```python
from build123d import *

# Parameters (mm, degrees)
SKETCH1_W           = 95
SKETCH1_H           = 75
BOSS_EXTRUDE1_DEPTH = 2
SKETCH2_W           = 14
SKETCH2_H           = 4
SKETCH2_W_2         = 13
BOSS_EXTRUDE2_DEPTH = 4
SKETCH3_W           = 12
SKETCH3_H           = 4
SKETCH3_W_2         = 11
BOSS_EXTRUDE3_DEPTH = 250
SKETCH4_W           = 10
SKETCH4_H           = 4
SKETCH4_W_2         = 9
BOSS_EXTRUDE4_DEPTH = 4
SKETCH5_W           = 4
SKETCH5_H           = 15
BOSS_EXTRUDE5_DEPTH = 4
SKETCH6_W           = 20
SKETCH6_H           = 4
BOSS_EXTRUDE6_DEPTH = 4


with BuildPart() as part:
    # Sketch1 → Boss-Extrude1 (new, symmetric)
    with BuildSketch(Plane.XY):
        Rectangle(SKETCH1_W, SKETCH1_H)
    extrude(amount=BOSS_EXTRUDE1_DEPTH, both=True)

    # Sketch2 → Boss-Extrude2 (add)
    with BuildSketch(Plane(origin=(0, 37.5, 0), x_dir=(1, 0, 0), z_dir=(0, 1, 0))):
        with Locations((40.5, 0)):
            Rectangle(SKETCH2_W, SKETCH2_H)
        with Locations((21, 0)):
            Rectangle(SKETCH2_W_2, SKETCH2_H)
        with Locations((-40.5, 0)):
            Rectangle(SKETCH2_W, SKETCH2_H)
        with Locations((-21, 0)):
            Rectangle(SKETCH2_W_2, SKETCH2_H)
    extrude(amount=BOSS_EXTRUDE2_DEPTH)

    # Sketch3 → Boss-Extrude3 (add)
    with BuildSketch(Plane(origin=(0, 41.5, 0), x_dir=(1, 0, 0), z_dir=(0, 1, 0))):
        with Locations((41.5, 0)):
            Rectangle(SKETCH3_W, SKETCH3_H)
        with Locations((22, 0)):
            Rectangle(SKETCH3_W_2, SKETCH3_H)
        with Locations((-22, 0)):
            Rectangle(SKETCH3_W_2, SKETCH3_H)
        with Locations((-41.5, 0)):
            Rectangle(SKETCH3_W, SKETCH3_H)
    extrude(amount=BOSS_EXTRUDE3_DEPTH)

    # Sketch4 → Boss-Extrude4 (add)
    with BuildSketch(Plane(origin=(0, 291.5, 0), x_dir=(1, 0, 0), z_dir=(0, 1, 0))):
        with Locations((-42.5, 0)):
            Rectangle(SKETCH4_W, SKETCH4_H)
        with Locations((-21, 0)):
            Rectangle(SKETCH4_W_2, SKETCH4_H)
        with Locations((21, 0)):
            Rectangle(SKETCH4_W_2, SKETCH4_H)
        with Locations((42.5, 0)):
            Rectangle(SKETCH4_W, SKETCH4_H)
    extrude(amount=BOSS_EXTRUDE4_DEPTH)

    # Sketch5 → Boss-Extrude5 (add)
    with BuildSketch(Plane.ZY.offset(47.5)):
        with Locations((0, -15)):
            Rectangle(SKETCH5_W, SKETCH5_H)
        with Locations((0, 15)):
            Rectangle(SKETCH5_W, SKETCH5_H)
    extrude(amount=BOSS_EXTRUDE5_DEPTH)

    # Sketch6 → Boss-Extrude6 (add)
    with BuildSketch(Plane.XZ.offset(37.5)):
        with Locations((-35.5, 0)):
            Rectangle(SKETCH6_W, SKETCH6_H)
        with Locations((35.5, 0)):
            Rectangle(SKETCH6_W, SKETCH6_H)
        Rectangle(SKETCH6_W, SKETCH6_H)
    extrude(amount=BOSS_EXTRUDE6_DEPTH)


solid = part.part
```
Could you check a few things on this model? Use its own coordinates, in mm. Coordinates: 2 decimals unless noted, no trailing zeros. Write each loop counter-clockwise with the first axis right and the second up, starting at its lowest first coordinate (ties: lowest second). Pieces come first, ordered by that corner, then holes. Notation, with made-up numbers: (-2.75, 36) - (13.25, 36) arc R32 cw to (13.25, 72) - close; hole circle Ø6 at (34, 32). An arc over 180 degrees is marked (long way). Use a Markdown table: item, result.
Q1. Imagine slicing it at A-A (y = 120). List the corners of the cut face in (x, z) for me, and give its area (3 significant figures).
Geometry check:
| item | result |
|---|---|
| outline | (-47.5, -2) - (-35.5, -2) - (-35.5, 2) - (-47.5, 2) - close; (-27.5, -2) - (-16.5, -2) - (-16.5, 2) - (-27.5, 2) - close; (16.5, -2) - (27.5, -2) - (27.5, 2) - (16.5, 2) - close; (35.5, -2) - (47.5, -2) - (47.5, 2) - (35.5, 2) - close |
| area | 184 mm2 |
Q2. I'm going to push flat-ended pins straight in: pin 1 Ø2 at (y, z) = (-39.5, 0.5) entering from +X; pin 2 Ø0.6 at (x, z) = (-15.5, 0) entering from +Y; pin 3 Ø2 at (x, z) = (-20.5, 0) entering from -Y. Where does each tip first touch, or does it pass through?
Geometry check:
| item | result |
|---|---|
| pin 1 | stops at x = 45.5 |
| pin 2 | stops at y = 41.5 |
| pin 3 | stops at y = -37.5 |
Q3. Please list where these lines run through material, in increasing order: L1, parallel to X at y = 225.5, z = 0.75; L2, parallel to Y at x = 24, z = 0.15; L3, parallel to Y at x = 32.5, z = 0.7.
Geometry check:
| item | result |
|---|---|
| L1 | x = -47.5 to -35.5, -27.5 to -16.5, 16.5 to 27.5, 35.5 to 47.5 |
| L2 | y = -37.5 to 295.5 |
| L3 | y = -41.5 to 37.5 |
Q4. Imagine slicing it at B-B (x = 2). List the corners of the cut face in (y, z) for me, and give its area (3 significant figures).
Geometry check:
| item | result |
|---|---|
| outline | (-41.5, -2) - (37.5, -2) - (37.5, 2) - (-41.5, 2) - close |
| area | 316 mm2 |
